```python
from build123d import *

# Parameters (mm, degrees)
SKETCH_R        = 62.5
PAD_DEPTH       = 100
PAD_TAPER       = 15
SKETCH001_R     = 50
PAD001_DEPTH    = 180
SKETCH002_R     = 50
PAD002_DEPTH    = 180
SKETCH003_R     = 47
POCKET_DEPTH    = 233.196381
SKETCH004_R     = 47
POCKET001_DEPTH = 233.196381
SKETCH005_R     = 59.5
POCKET002_DEPTH = 75
POCKET002_TAPER = 15
PAD003_DEPTH    = 20
POCKET003_DEPTH = 20


with BuildPart() as part:
    # Sketch → Pad (new body)
    with BuildSketch(Plane.XY):
        Circle(SKETCH_R)
    extrude(amount=PAD_DEPTH, taper=PAD_TAPER)

    # Sketch001 (on DatumPlane) → Pad001 (join)
    with BuildSketch(Plane(origin=(0, 0, 0), x_dir=(1, 0, 0), z_dir=(0, 0.34202, 0.939693))):
        Circle(SKETCH001_R)
    extrude(amount=PAD001_DEPTH)

    # Sketch002 (on DatumPlane) → Pad002 (join)
    with BuildSketch(Plane(origin=(0, 0, 0), x_dir=(1, 0, 0), z_dir=(0, -0.34202, 0.939693))):
        Circle(SKETCH002_R)
    extrude(amount=PAD002_DEPTH)

    # Sketch003 (on Face7 of Pad002) → Pocket (cut, through all)
    with BuildSketch(Plane(origin=(0, 61.563626, 169.144672), x_dir=(1, 0, 0), z_dir=(0, 0.34202, 0.939693))):
        Circle(SKETCH003_R)
    extrude(amount=-POCKET_DEPTH, mode=Mode.SUBTRACT)

    # Sketch004 (on Face8 of Pocket) → Pocket001 (cut, through all)
    with BuildSketch(Plane(origin=(0, -61.563626, 169.144672), x_dir=(1, 0, 0), z_dir=(0, -0.34202, 0.939693))):
        Circle(SKETCH004_R)
    extrude(amount=-POCKET001_DEPTH, mode=Mode.SUBTRACT)

    # Sketch005 (on Face2 of Pocket001) → Pocket002 (cut)
    with BuildSketch(Plane(origin=(0, 0, 0), x_dir=(1, 0, 0), z_dir=(0, 0, -1))):
        Circle(SKETCH005_R)
    extrude(amount=-POCKET002_DEPTH, taper=POCKET002_TAPER, mode=Mode.SUBTRACT)

    # Sketch → Pad003 (join)
    with BuildSketch(Plane.XY):
        Circle(SKETCH_R)
    extrude(amount=-PAD003_DEPTH)

    # Sketch005 (on Face2 of Pocket001) → Pocket003 (cut)
    with BuildSketch(Plane(origin=(0, 0, 0), x_dir=(1, 0, 0), z_dir=(0, 0, -1))):
        Circle(SKETCH005_R)
    extrude(amount=POCKET003_DEPTH, mode=Mode.SUBTRACT)


solid = part.part
```
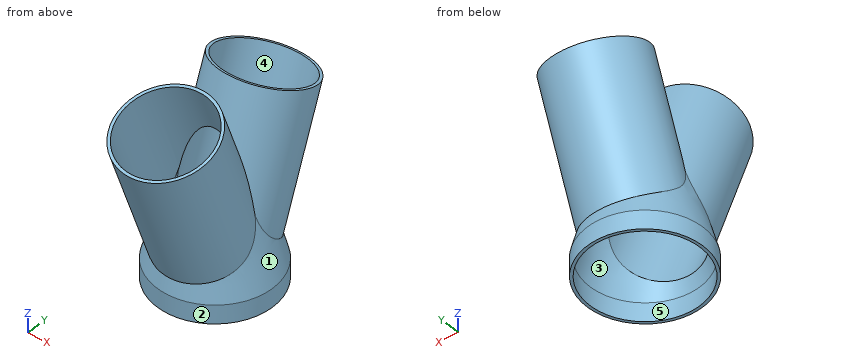
Design review of the part built by this model. Coordinates are the model's own, in mm. Face numbers are marked on the shaded views. A direction names the side the tool comes from. Give positions to 0.01 mm unless a question says otherwise; leave off trailing zeros. Write each loop counter-clockwise with the first axis right and the second up, starting at its lowest first coordinate (ties: lowest second). Pieces come first, ordered by that corner, then holes. Notation, with made-up numbers: (-28.5, 8.25) - (18.5, 8.25) arc R19 cw to (18.5, 42.25) - close; hole circle Ø4 at (5, 7.25). An arc over 180 degrees is marked (long way). Return JSON: item names as keys, results as strings. Group by question number.
(1) We need section B-B, the plane x = 18. Give the number of separate pieces and of enclosed holes in the cut face, then the cut area to 3 significant figures.
(2) To check wall thickness, follow probe 1 along Y at (x, z) = (1, -11); probe 2 along X at (y, z) = (-32.5, 177); probe 3 along Y at (x, z) = (-40, 2.5). State the ranges of each line that lie inside material, in increasing order.
(3) Mouldability with a two-part tool opening along Z and no side actions: class the marked faces 3, 4 and 5 as +Z half, -Z half, draft (parallel to the pull), parting line (faces both ways), or undercut.
(4) Machinability: for the marked faces 1 and 2, which of the approach directions +Z, -Z, +X, -X, +Y, -Y give a long, thin tool a straight path to every point of the face, cutting with its end or side? Answer none if there is none.
(5) Insertion check: pin 1 (6 mm diameter, centred on y = 16, z = 57, fed in from -X); pin 2 (1.5 mm diameter, centred on y = 36, z = 79, fed in from +X); pin 3 (2 mm diameter, centred on x = -32, z = 63, fed in from +Y). Each pin has a flat end and moves straight along its axis. Give the tip position at first contact, or say it passes through.
(6) We need section A-A, the plane x = 0. Give the boundary of the cut face in (y, z).
Reported:
{
 "1": {"separate pieces": "3", "enclosed holes": "0", "area": "1,540 mm2"},
 "2": {"probe 1": "y = -62.49 to -59.49, 59.49 to 62.49", "probe 2": "x = -40 to -36.18, 36.18 to 40", "probe 3": "y = -47.15 to -43.14, 43.14 to 47.15"},
 "3": {"face 3": "-Z half", "face 4": "undercut", "face 5": "draft"},
 "4": {"face 1": "none", "face 2": "-Z"},
 "5": {"pin 1": "stops at x = -49.98", "pin 2": "stops at x = 49.63", "pin 3": "stops at y = 64.75"},
 "6": {"outline": "(-108.55, 152.04) - (-58.56, 14.7) - (-62.5, 0) - (-62.5, -20) - (-59.5, -20) - (-59.5, 0) - (-55.48, 15.01) - (-105.73, 153.07) - close; (-17.4, 185.22) - (0, 137.42) - (17.4, 185.22) - (14.58, 186.25) - (0, 146.19) - (-14.58, 186.25) - close; (55.48, 15.01) - (59.5, 0) - (59.5, -20) - (62.5, -20) - (62.5, 0) - (58.56, 14.7) - (108.55, 152.04) - (105.73, 153.07) - close"}
}
